from build123d import *

# Parameters (mm, degrees)
SKETCH_1_R      = 9
SKETCH_1_R_2    = 8
EXTRUDE_1_DEPTH = 3
FILLET_1_R      = 0.25


with BuildPart() as part:
    # 草图1 → 凸台-拉伸1 (new body)
    with BuildSketch(Plane(origin=(0, 0, 0), x_dir=(1, 0, 0), z_dir=(0, 1, 0))):
        Circle(SKETCH_1_R)
        Circle(SKETCH_1_R_2, mode=Mode.SUBTRACT)
    extrude(amount=EXTRUDE_1_DEPTH)

    # 圆角1
    fillet_1_edges = [part.edges().sort_by_distance(p)[0] for p in [
        (-9, 0, 0),
        (-8, 0, 0),
        (-8, 3, 0),
    ]]
    fillet(fillet_1_edges, radius=FILLET_1_R)


solid = part.part
The listing builds one solid part. Answer for the finished solid, in the listing's coordinates (mm). Give positions to 0.01 mm unless a question says otherwise; leave off trailing zeros. Loops run counter-clockwise (first coordinate to the right, second up) from the corner with the lowest first, then second, coordinate; pieces in that order, holes last. Notation, with made-up numbers: (68.25, 61) - (110.25, 61) arc R22 cw to (110.25, 91) - close; hole circle Ø6 at (25, 60). An arc over 180 degrees is marked (long way). Answer as a JSON object with one key per item and string values.
1. Find the intervals of material crossed by L1, parallel to Z at x = 0, y = 1.6; L2, parallel to X at y = 2.85, z = -6, in increasing order. Write a range as [from, to].
Determined:
{"L1": "[-9, -8], [8, 9]", "L2": "[-6.71, -5.32], [5.32, 6.71]"}
2. For a pull along X with two mould halves and no side action, classify faces 1 (the cylindrical face through (-1.73, 1.48, 7.81)), 2 (the cylindrical face through (-1.172, 1.606, -8.923)), 3 (the flat face through (8, 3, 3)) as pulls with the +X half, pulls with the -X half, needs draft (parallel to the pull), parting line crosses it, or undercut.
Determined:
{"face 1": "undercut", "face 2": "parting line crosses it", "face 3": "needs draft"}
3. A cutting plane is placed at C-C (y = 0.8). Write down the section's boundary in (x, z).
Determined:
{"outline": "circle Ø18 at (0, 0); hole circle Ø16 at (0, 0)"}
4. A cutting plane is placed at A-A (z = 0). Write down the section's boundary in (x, y).
Determined:
{"outline": "(-9, 0.25) arc R0.25 ccw to (-8.75, 0) - (-8.25, 0) arc R0.25 ccw to (-8, 0.25) - (-8, 2.75) arc R0.25 ccw to (-8.25, 3) - (-9, 3) - close; (8, 0.25) arc R0.25 ccw to (8.25, 0) - (8.75, 0) arc R0.25 ccw to (9, 0.25) - (9, 3) - (8.25, 3) arc R0.25 ccw to (8, 2.75) - close"}
5. A cutting plane is placed at B-B (x = 0). Write down the section's boundary in (y, z), then the cut area to 3 significant figures.
Determined:
{"outline": "(0, -8.75) arc R0.25 ccw to (0.25, -9) - (3, -9) - (3, -8.25) arc R0.25 ccw to (2.75, -8) - (0.25, -8) arc R0.25 ccw to (0, -8.25) - close; (0, 8.25) arc R0.25 ccw to (0.25, 8) - (2.75, 8) arc R0.25 ccw to (3, 8.25) - (3, 9) - (0.25, 9) arc R0.25 ccw to (0, 8.75) - close", "area": "5.92 mm²"}
6. Flat-ended cylindrical pins translate along their axes: pin 1 Ø10 at (x, z) = (-0.5, -0.5) entering from -Y; pin 2 Ø1 at (x, y) = (-5.5, 2) entering from +Z; pin 3 Ø1.5 at (y, z) = (0.5, 1) entering from +X. Find the tip coordinate at first contact, or state that the pin passes through.
Determined:
{"pin 1": "through", "pin 2": "z = 7.48", "pin 3": "x = 9"}
